Work out the finished part from the listing and answer in its coordinate system (mm). A direction names the side the tool comes from. Coordinates: 2 decimals unless noted, no trailing zeros. Order: outer loops, then holes, each group sorted by start corner. A loop starts at its lowest first (then second) coordinate and runs counter-clockwise, first axis right, second up. Notation, with made-up numbers: (71, 38.25) -> (96, 38.25) arc R22 cw to (96, 59.25) -> close; hole circle Ø8 at (77, 24). An arc over 180 degrees is marked (long way). Write item = value, one per line. Start each with the question number.
Q1. Straight lines are drawn through the part: L1, parallel to Y at x = 42, z = -0.1; L2, parallel to Y at x = 48.5, z = 0.3; L3, parallel to Z at x = 15.5, y = 15. For each, find the intervals that lie inside material, in ascending order. Write a range as from..to.
Q2. Flat-ended cylindrical pins translate along their axes: pin 1 (4 mm diameter, centred on x = 50.24, y = 24, fed in from -Z); pin 2 (0.5 mm diameter, centred on y = 0, z = -0.5, fed in from -X); pin 3 (0.8 mm diameter, centred on y = -4.5, z = -0.5, fed in from +X). Find the tip coordinate at first contact, or state that the pin passes through.
Q3. For a pull along X with two mould halves and no side action, classify faces 1 (the cylindrical face through (-52.65, 0.33, 2.56)), 2 (the cylindrical face through (48.108, 23.328, 0.406)), 3 (the cylindrical face through (-0.69, 26.4, 2.56)) as +X half, -X half, draft (parallel to the pull), parting line (faces both ways), or undercut.
Q4. The part is cut by section B-B, the plane x = -13. Determine the outline of the cut face in (y, z).
Q5. The part is cut by section A-A, the plane y = -15.5. Determine the outline of the cut face in (x, z).
Q6. Which of the six approach directions +Z, -Z, +X, -X, +Y, -Y give full straight-line access (tool end or side, diameter ignored) to faces 4 (the flat face through (-1, 0, 3.5)), 5 (the cylindrical face through (-52.316, -23.146, 0.406))?
```python
from build123d import *

# Parameters (mm, degrees)
F1_DEPTH     = 3.5
F5_D         = 4.473
F5_DEPTH     = 0.8
F5_TIP       = 1.3438247745
F6_T1_DEPTH  = 99
F6_T3_DEPTH  = 46.5
F6_T6_ANGLE  = 90
F6_T8_ANGLE  = 90
F6_T10_ANGLE = 90
F6_T12_ANGLE = 90
F8_W         = 0.5
F8_H         = 37.5
F8_W_2       = 88
F8_H_2       = 0.5
F9_DEPTH     = 1


# Not quite as in the source:
# - a fillet or chamfer that OpenCascade refuses, or shapes differently, is made with other operations: its cross-section is extruded or revolved along the edge and cut away or added


with BuildPart() as f1:
    # F0 (on Top) → F1 (new body)
    with BuildSketch(Plane.XY):
        with BuildLine():
            Line((-49.5, -28.25), (49.5, -28.25))
            ThreePointArc((49.5, -28.25), (53.0355339059, -26.7855339059), (54.5, -23.25))
            Line((54.5, -23.25), (54.5, 23.25))
            ThreePointArc((54.5, 23.25), (53.0355339059, 26.7855339059), (49.5, 28.25))
            Line((49.5, 28.25), (-49.5, 28.25))
            ThreePointArc((-49.5, 28.25), (-53.0355339059, 26.7855339059), (-54.5, 23.25))
            Line((-54.5, 23.25), (-54.5, -23.25))
            ThreePointArc((-54.5, -23.25), (-53.0355339059, -26.7855339059), (-49.5, -28.25))
        make_face()
    extrude(amount=F1_DEPTH)

    # F5
    with Locations(Plane(origin=(0, 0, 0), x_dir=(1, 0, 0), z_dir=(0, 0, -1))):
        with Locations((-50.2406740561, -23.9985361695), (-50.2495961264, 24.0030474961), (50.2488752827, 23.995583877), (50.2413948998, -24.0000952035)):
            Hole(F5_D / 2, depth=F5_DEPTH)
            with Locations((0, 0, -(F5_DEPTH + F5_TIP / 2))):  # 118° drill point
                Cone(0, F5_D / 2, F5_TIP, mode=Mode.SUBTRACT)

    # F6: fillet of radius 5 on 1 edges, made by hand

    # F6_s2 → F6_t1 (cut)
    with BuildSketch(Plane.YZ.offset(-49.5)):
        with BuildLine():
            ThreePointArc((-28.25, 0), (-26.4383438845, 2.5311288741), (-23.4803039929, 3.5))
            Line((-23.4803039929, 3.5), (-28.25, 3.5))
            Line((-28.25, 3.5), (-28.25, 0))
        make_face()
        with BuildLine():
            ThreePointArc((23.4803039929, 3.5), (26.4383438845, 2.5311288741), (28.25, 0))
            Line((28.25, 0), (28.25, 3.5))
            Line((28.25, 3.5), (23.4803039929, 3.5))
        make_face()
    extrude(amount=F6_T1_DEPTH, mode=Mode.SUBTRACT)

    # F6_s4 → F6_t3 (cut)
    with BuildSketch(Plane.XZ.offset(-23.25)):
        with BuildLine():
            ThreePointArc((49.7303039929, 3.5), (52.6883438845, 2.5311288741), (54.5, 0))
            Line((54.5, 0), (54.5, 3.5))
            Line((54.5, 3.5), (49.7303039929, 3.5))
        make_face()
        with BuildLine():
            ThreePointArc((-49.7303039929, 3.5), (-52.6883438845, 2.5311288741), (-54.5, 0))
            Line((-54.5, 0), (-54.5, 3.5))
            Line((-54.5, 3.5), (-49.7303039929, 3.5))
        make_face()
    extrude(amount=F6_T3_DEPTH, mode=Mode.SUBTRACT)

    # F6_s5 → F6_t6 (revolve, cut)
    with BuildSketch(Plane.XZ.offset(23.25)):
        with BuildLine():
            ThreePointArc((-54.5, 0), (-52.6883438845, 2.5311288741), (-49.7303039929, 3.5))
            Line((-49.7303039929, 3.5), (-54.5, 3.5))
            Line((-54.5, 3.5), (-54.5, 0))
        make_face()
    revolve(axis=Axis((-49.5, -23.25, 3.5), (0, 0, 1)), revolution_arc=F6_T6_ANGLE, mode=Mode.SUBTRACT)

    # F6_s7 → F6_t8 (revolve, cut)
    with BuildSketch(Plane.YZ.offset(49.5)):
        with BuildLine():
            ThreePointArc((-28.25, 0), (-26.4383438845, 2.5311288741), (-23.4803039929, 3.5))
            Line((-23.4803039929, 3.5), (-28.25, 3.5))
            Line((-28.25, 3.5), (-28.25, 0))
        make_face()
    revolve(axis=Axis((49.5, -23.25, 3.5), (0, 0, 1)), revolution_arc=F6_T8_ANGLE, mode=Mode.SUBTRACT)

    # F6_s9 → F6_t10 (revolve, cut)
    with BuildSketch(Plane.XZ.offset(-23.25)):
        with BuildLine():
            ThreePointArc((49.7303039929, 3.5), (52.6883438845, 2.5311288741), (54.5, 0))
            Line((54.5, 0), (54.5, 3.5))
            Line((54.5, 3.5), (49.7303039929, 3.5))
        make_face()
    revolve(axis=Axis((49.5, 23.25, 3.5), (0, 0, 1)), revolution_arc=F6_T10_ANGLE, mode=Mode.SUBTRACT)

    # F6_s11 → F6_t12 (revolve, cut)
    with BuildSketch(Plane.YZ.offset(-49.5)):
        with BuildLine():
            ThreePointArc((23.4803039929, 3.5), (26.4383438845, 2.5311288741), (28.25, 0))
            Line((28.25, 0), (28.25, 3.5))
            Line((28.25, 3.5), (23.4803039929, 3.5))
        make_face()
    revolve(axis=Axis((-49.5, 23.25, 3.5), (0, 0, 1)), revolution_arc=F6_T12_ANGLE, mode=Mode.SUBTRACT)

    # F8 (on Top) → F9 (join)
    with BuildSketch(Plane.XY):
        with Locations((-53.0630070642, -0.0139670707)):
            Rectangle(F8_W, F8_H)
        with Locations((-0.0016481951, -26.7570052035)):
            Rectangle(F8_W_2, F8_H_2)
        with Locations((53.0663034543, -0.0139678158)):
            Rectangle(F8_W, F8_H)
        with Locations((-0.0016481951, 26.78494009)):
            Rectangle(F8_W_2, F8_H_2)
    extrude(amount=-F9_DEPTH)


solid = f1.part
```
Model answer:
q1.L1 = -27.01..-26.51, 26.53..27.03
q1.L2 = -28.15..-25.39, -22.6..22.6, 25.4..28.15
q1.L3 = 0..3.5
q2.pin_1 = 0.94
q2.pin_2 = -53.31
q2.pin_3 = 53.32
q3.face_1 = -X half
q3.face_2 = undercut
q3.face_3 = draft
q4.outline = (-28.25, 0) -> (-27.01, 0) -> (-27.01, -1) -> (-26.51, -1) -> (-26.51, 0) -> (26.53, 0) -> (26.53, -1) -> (27.03, -1) -> (27.03, 0) -> (28.25, 0) arc R5 ccw to (23.48, 3.5) -> (-23.48, 3.5) arc R5 ccw to start
q5.outline = (-54.5, 0) -> (-53.31, 0) -> (-53.31, -1) -> (-52.81, -1) -> (-52.81, 0) -> (52.82, 0) -> (52.82, -1) -> (53.32, -1) -> (53.32, 0) -> (54.5, 0) arc R5 ccw to (49.73, 3.5) -> (-49.73, 3.5) arc R5 ccw to start
q6.face_4 = +Z, +X, -X, +Y, -Y
q6.face_5 = -Z
